Geometry check sheet. Reference: the model listing, model coordinates, mm. A direction names the side the tool comes from. Give positions to 0.01 mm unless a question says otherwise; leave off trailing zeros. Write each loop counter-clockwise with the first axis right and the second up, starting at its lowest first coordinate (ties: lowest second). Pieces come first, ordered by that corner, then holes. Notation, with made-up numbers: (-36.75, 18) - (-26.75, 18) arc R33 cw to (-26.75, 46) - close; hole circle Ø8 at (-5.75, 23). An arc over 180 degrees is marked (long way). Write item = value, one per line. Start each with the question number.
(1) Section check B-B, the plane y = 1.5. Enter the section's corners in (x, z), plus the area to 3 significant figures.
(2) Draft check along X on faces 1 (the flat face through (-10, 0, 153)), 2 (the flat face through (8.749, 0.14, 0.213)), 3 (the flat face through (-8, 0, 153)), 4 (the flat face through (10, 0, 153)). Enter one of: pulls with the +X half, pulls with the -X half, needs draft (parallel to the pull), parting line crosses it, or undercut.
(3) Section check C-C, the plane z = 171. Enter the section's corners in (x, y).
(4) Access from +Z, -Z, +X, -X, +Y, -Y to the whole of each face (thin tool, end or side, straight path). Record for faces 5 (the flat face through (0, 8, 153)), 6 (the flat face through (0, 10, 153)).
(5) Thickness scan on L1, parallel to Y at x = -2.25, z = 79; L2, parallel to X at y = -7.5, z = 166.5. Record the ranges inside material, lowest first.
Autodesk Inventor part; units mm, degrees
ref_plane "Start Plane" through (0, 0, -9.7168) normal (0, 0, 1) x (1, 0, 0)
ref_plane "End Plane" through (0, 0, 319.7611) normal (0, 0, 1) x (1, 0, 0)
ref_plane "Work Plane4" through (0, 10.1778, 319.941) normal (0, -0.7112, 0.703) x (1, 0, 0)
ref_plane "Start Plane" through (0, 0, -9.7168) normal (0, 0, 1) x (1, 0, 0)
ref_plane "End Plane" through (0, 0, 319.7611) normal (0, 0, 1) x (1, 0, 0)
sketch "Sketch" plane through (0, 0, 0) normal (0, 0, 1) x (1, 0, 0)
  line L0 (-10, -7) -> (-10, 7)
  line L1 (-7, 10) -> (7, 10)
  line L2 (10, 7) -> (10, -7)
  line L3 (7, -10) -> (-7, -10)
  arc A0 (-10, -7) -> (-7, -10) centre (-7, -7) ccw
  arc A1 (-7, 10) -> (-10, 7) centre (-7, 7) ccw
  arc A2 (10, 7) -> (7, 10) centre (7, 7) ccw
  arc A3 (7, -10) -> (10, -7) centre (7, -7) ccw
  arc A4 (-7, 8) -> (-8, 7) centre (-7, 7) ccw
  line L4 (-7, 8) -> (7, 8)
  arc A5 (8, 7) -> (7, 8) centre (7, 7) ccw
  line L5 (8, 7) -> (8, -7)
  arc A6 (7, -8) -> (8, -7) centre (7, -7) ccw
  line L6 (7, -8) -> (-7, -8)
  arc A7 (-8, -7) -> (-7, -8) centre (-7, -7) ccw
  line L7 (-8, -7) -> (-8, 7)
  line L8 (0, 14.8698) -> (0, -14.8698) construction
  line L9 (-14.8698, 0) -> (14.8698, 0) construction
  dimension "d7" = 3
  dimension "d10" = 20
  dimension "d11" = 20
  dimension "d12" = 2
  dimension "d15" = 10
  dimension "d16" = 10
extrude "Body" add sketch "Sketch" along normal up to surface (329.478 mm away) from surface at -9.7168
sketch "Sketch3" plane through (0, 0, 0) normal (0, 0, 1) x (1, 0, 0)
  line L0 (0, 0) -> (10, 0)
ref_plane "Work Plane3" through (0, 0, 0) normal (0, -1, 0) x (1, 0, 0)
sketch "Sketch4" plane through (0, 0, 0) normal (0, -1, 0) x (1, 0, 0)
  line L0 (-2, -9.7168) -> (12, -9.7168)
  line L1 (-2, 319.7611) -> (12, 319.7611)
  dimension "d18" = 329.478
ref_plane "Work Plane4" through (0, 10.1778, 319.941) normal (0, -0.7112, 0.703) x (1, 0, 0)
split "Split1" plane through (0, 10.1778, 319.941) removes the side toward (0, -0.7112, 0.703)
ref_plane "Work Plane5" through (0, 10.1774, -9.8955) normal (0, -0.7096, -0.7046) x (1, 0, 0)
split "Split2" plane through (0, 10.1774, -9.8955) removes the side toward (0, -0.7096, -0.7046)
equation "\"d7\" = G_IR"
equation "\"d10\" = G_H"
equation "\"d11\" = G_W"
equation "\"d12\" = G_T"
equation "\"d15\" = 0.5 * d10"
equation "\"d16\" = 0.5 * d11"
equation "\"d3\" = G_L"
equation "\"G_W\" = 20"
equation "\"G_H\" = 20"
equation "\"G_T\" = 2"
equation "\"G_IR\" = 3"
equation "\"G_L\" = d18"
equation "\"G_OFFSET_START\" = 9.71683"
equation "\"G_OFFSET_END\" = 9.76112"
equation "\"d13\" = -G_OFFSET_START"
equation "\"d14\" = G_OFFSET_END + B_L"
properties part number "ISO 12633-2 - 20x20x2 - 329.48" material "Steel, Mild"
Model answer:
q1.outline = (-10, -1.16) - (-8, -1.16) - (-8, 311.16) - (-10, 311.16) - close; (8, -1.16) - (10, -1.16) - (10, 311.16) - (8, 311.16) - close
q1.area = 1,250 mm²
q2.face_1 = pulls with the -X half
q2.face_2 = needs draft
q2.face_3 = undercut
q2.face_4 = pulls with the +X half
q3.outline = (-10, -7) arc R3 ccw to (-7, -10) - (7, -10) arc R3 ccw to (10, -7) - (10, 7) arc R3 ccw to (7, 10) - (-7, 10) arc R3 ccw to (-10, 7) - close; hole (-8, -7) arc R1 ccw to (-7, -8) - (7, -8) arc R1 ccw to (8, -7) - (8, 7) arc R1 ccw to (7, 8) - (-7, 8) arc R1 ccw to (-8, 7) - close
q4.face_5 = +Z, -Z
q4.face_6 = +Z, -Z, +X, -X, +Y
q5.L1 = -10 to -8, 8 to 10
q5.L2 = -9.96 to -7.87, 7.87 to 9.96
